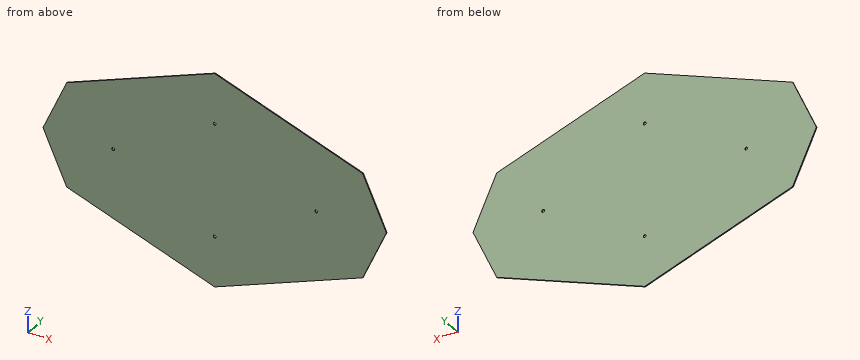
from build123d import *

# Parameters (mm, degrees)
BOSS_EXTRUDE1_DEPTH   = 1.190625
SKETCH2_R             = 3.175
CUT_EXTRUDE1_DEPTH    = 456.240158496
CRVPATTERN1_START     = -1.190625
CRVPATTERN1_OUTLINE_R = 3.175
CRVPATTERN1_DEPTH     = 2.38125


# Read off the part's stored shape, not the designer's step: CrvPattern1
with BuildPart() as part:
    # Sketch1 → Boss-Extrude1 (new, symmetric)
    with BuildSketch(Plane(origin=(0, 0, 0), x_dir=(1, 0, 0), z_dir=(0, 1, 0))):
        Polygon((-333.074526413, 117.648642651), (0, 240.597926469), (333.074526413, 117.648642651), (386.459013784, 0), (333.074526413, -117.648642651), (0, -240.597926469), (-333.074526413, -117.648642651), (-386.459013784, 0), align=None)
    extrude(amount=BOSS_EXTRUDE1_DEPTH, both=True)

    # Sketch2 → Cut-Extrude1 (cut, through all)
    with BuildSketch(Plane(origin=(0, 1.190625, 0), x_dir=(1, 0, 0), z_dir=(0, 1, 0))):
        with Locations(Location((0, 127, 0), (0, 0, 270))):
            Circle(SKETCH2_R)
    extrude(amount=-CUT_EXTRUDE1_DEPTH, mode=Mode.SUBTRACT)

    # CrvPattern1 outline → CrvPattern1 (cut)
    with BuildSketch(Plane(origin=(0, 0, 0), x_dir=(1, 0, 0), z_dir=(0, 1, 0)).offset(CRVPATTERN1_START)):
        with Locations((-228.6, 0)):
            Circle(CRVPATTERN1_OUTLINE_R)
        with Locations((0, -127)):
            Circle(CRVPATTERN1_OUTLINE_R)
        with Locations((228.6, 0)):
            Circle(CRVPATTERN1_OUTLINE_R)
    extrude(amount=CRVPATTERN1_DEPTH, mode=Mode.SUBTRACT)


solid = part.part
Input: part model. Units: mm. Frame: model coordinates. Coordinates: 2 decimals unless noted, no trailing zeros. Loops run counter-clockwise (first coordinate to the right, second up) from the corner with the lowest first, then second, coordinate; pieces in that order, holes last.
Q1. Material intervals for line 1 (X direction, y = 0.5, z = 0) (3 decimals); line 2 (X direction, y = -0.3, z = -57.5); line 3 (Z direction, x = 297, y = 1.05) (3 decimals), sorted ascending.
Q2. Cut plane C-C (x = 36.5). Output: boundary loops of the cut face in (y, z), then the cut area to 3 significant figures.
Q3. Cut plane B-B (z = 87.5). Output: boundary loops of the cut face in (x, y).
Q4. Cut plane A-A (y = -0.75). Output: boundary loops of the cut face in (x, z) (3 decimals).
Q5. Contact query for a flat-ended pin moving along its axis: pin 1 (5 mm diameter, centred on x = 0, z = -127, fed in from +Y). Output: stop coordinate, or through.
Working result:
1. line 1: x = -386.459 to -231.775, -225.425 to 225.425, 231.775 to 386.459
1. line 2: x = -360.37 to 360.37
1. line 3: z = -130.965 to 130.965
2. outline: (-1.19, -227.12) - (1.19, -227.12) - (1.19, 227.12) - (-1.19, 227.12) - close
2. area: 1,080 mm2
3. outline: (-346.75, -1.19) - (346.75, -1.19) - (346.75, 1.19) - (-346.75, 1.19) - close
4. outline: (-386.459, 0) - (-333.075, -117.649) - (0, -240.598) - (333.075, -117.649) - (386.459, 0) - (333.075, 117.649) - (0, 240.598) - (-333.075, 117.649) - close; hole circle Ø6.35 at (-228.6, 0); hole circle Ø6.35 at (0, -127); hole circle Ø6.35 at (0, 127); hole circle Ø6.35 at (228.6, 0)
5. pin 1: passes through
